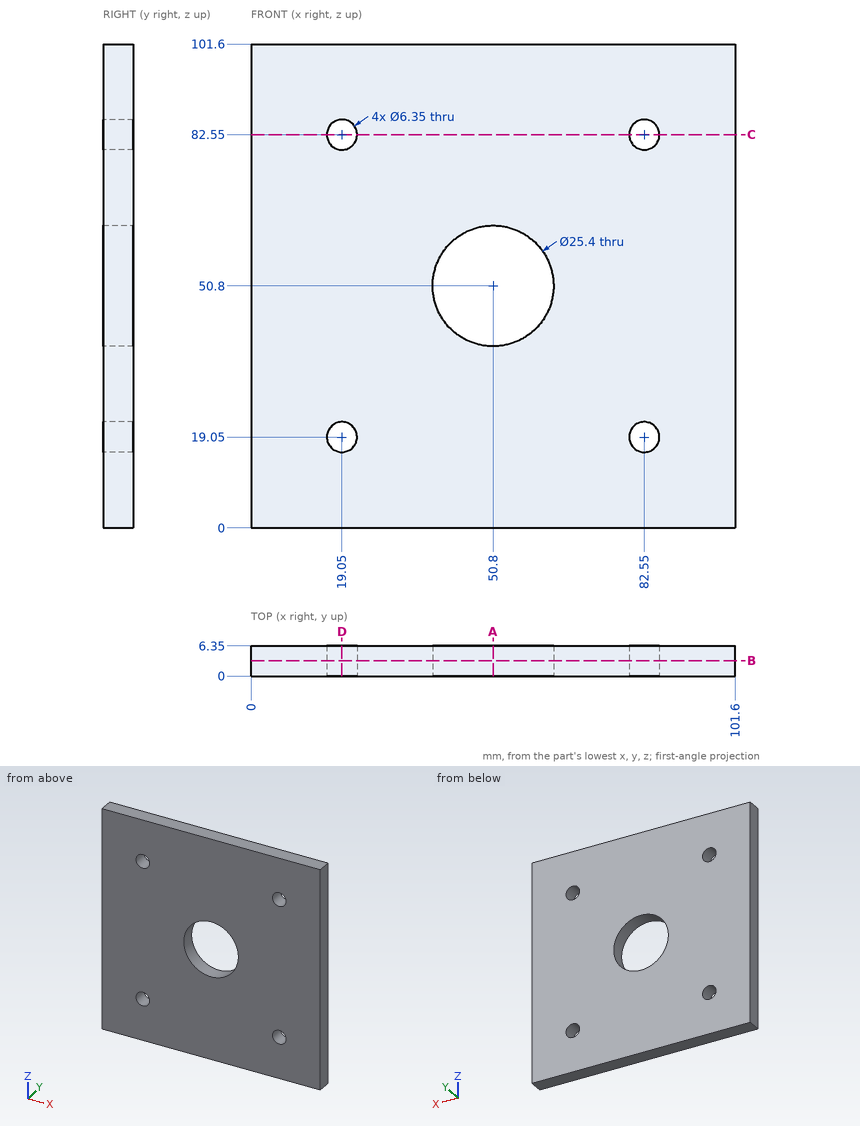
Answer from the drawing. Dimensions are ordinates in mm from the lowest x, y and z of the part. Coordinates: 2 decimals unless noted, no trailing zeros. Write each loop counter-clockwise with the first axis right and the second up, starting at its lowest first coordinate (ties: lowest second). Pieces come first, ordered by that corner, then holes. Notation, with made-up numbers: (54, -5.5) - (63, -5.5) arc R12 ccw to (63, 2.5) - close; hole circle Ø1 at (82.25, -22). An arc over 180 degrees is marked (long way). Answer as CSV lines item,"result".
1. Find section B-B (y = 3.25). Give the vertices of the cut face in (x, z) (3 decimals), plus the area to 3 significant figures.
Computed values:
outline,"(0, 0) - (101.6, 0) - (101.6, 101.6) - (0, 101.6) - close; hole circle Ø6.35 at (19.05, 19.05); hole circle Ø6.35 at (19.05, 82.55); hole circle Ø25.4 at (50.8, 50.8); hole circle Ø6.35 at (82.55, 19.05); hole circle Ø6.35 at (82.55, 82.55)"
area,"9,690 mm²"
2. Given P1, Ø5.5, axis at x = 82.55, z = 82.55, coming from the +Y side, flat-ended and moving along its own axis, determine where the tip first touches the part or whether it passes through.
Computed values:
P1,"passes through"
3. Find section C-C (z = 82.55). Give the vertices of the cut face in (x, y) (3 decimals).
Computed values:
outline,"(0, 0) - (15.875, 0) - (15.875, 6.35) - (0, 6.35) - close; (22.225, 0) - (79.375, 0) - (79.375, 6.35) - (22.225, 6.35) - close; (85.725, 0) - (101.6, 0) - (101.6, 6.35) - (85.725, 6.35) - close"
4. Find section D-D (x = 19.05). Give the vertices of the cut face in (y, z) (3 decimals), plus the area to 3 significant figures.
Computed values:
outline,"(0, 0) - (6.35, 0) - (6.35, 15.875) - (0, 15.875) - close; (0, 22.225) - (6.35, 22.225) - (6.35, 79.375) - (0, 79.375) - close; (0, 85.725) - (6.35, 85.725) - (6.35, 101.6) - (0, 101.6) - close"
area,"565 mm²"
5. Straight lines are drawn through the part: line 1 (X direction, y = 3.5, z = 82.55) (3 decimals); line 2 (Z direction, x = 21, y = 4.5). For each, find the intervals that lie inside material, in ascending order. Write a range as [from, to].
Computed values:
line 1,"x = [0, 15.875], [22.225, 79.375], [85.725, 101.6]"
line 2,"z = [0, 16.54], [21.56, 80.04], [85.06, 101.6]"
6. Find section A-A (x = 50.8). Give the vertices of the cut face in (y, z), plus the area to 3 significant figures.
Computed values:
outline,"(0, 0) - (6.35, 0) - (6.35, 38.1) - (0, 38.1) - close; (0, 63.5) - (6.35, 63.5) - (6.35, 101.6) - (0, 101.6) - close"
area,"484 mm²"
